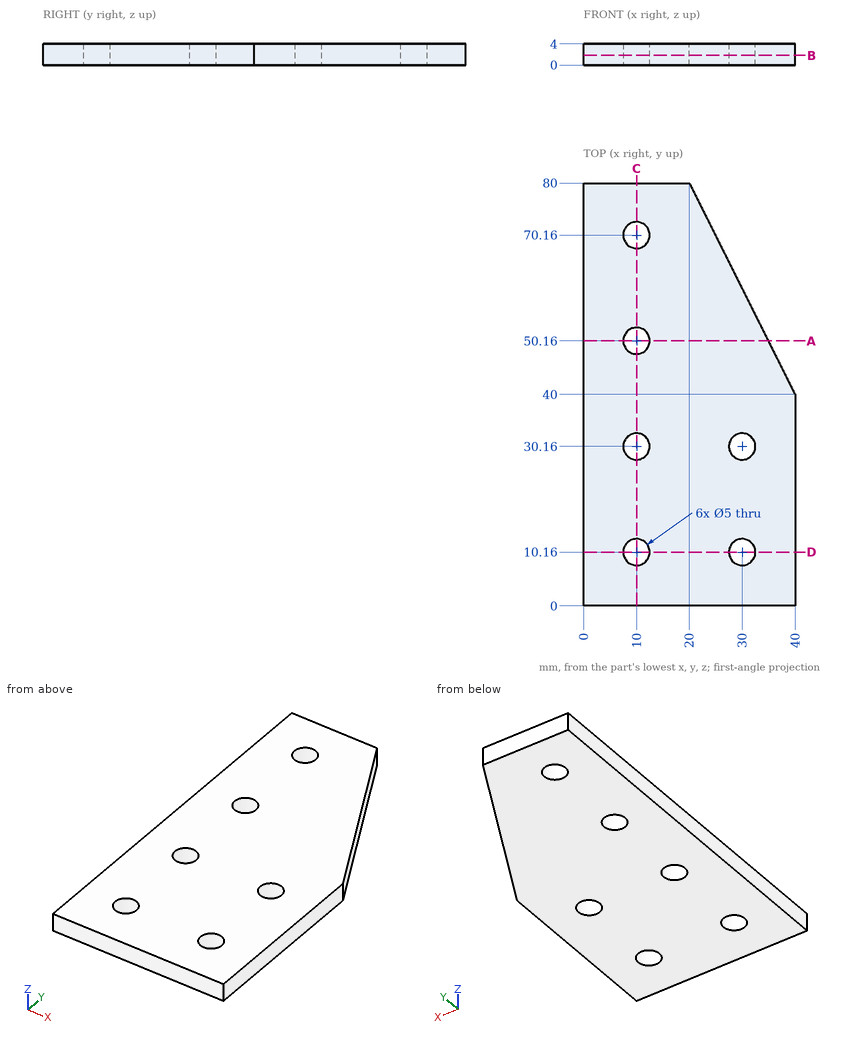
Verification items for this drawing (mm, ordinates from the low corner). Coordinates: 2 decimals unless noted, no trailing zeros. Write each loop counter-clockwise with the first axis right and the second up, starting at its lowest first coordinate (ties: lowest second). Pieces come first, ordered by that corner, then holes. Notation, with made-up numbers: M 43.5,32 L 86.5,32 A11 ccw 86.5,52 Z; hole C 43.5,43.5 d3. An arc over 180 degrees is marked long. Use CSV: the item, a comma, the result in double quotes.
Q1. Section check A-A, the plane y = 50.16. Enter the section's corners in (x, z).
Computed values:
outline,"M 0,0 L 7.5,0 L 7.5,4 L 0,4 Z; M 12.5,0 L 34.92,0 L 34.92,4 L 12.5,4 Z"
Q2. Thickness scan on line 1 along Y through (x, z) = (12, 2); line 2 along Y through (x, z) = (9, 0.3); line 3 along Y through (x, z) = (29, 1.65). Record the ranges inside material, lowest first. Write a range as [from, to].
Computed values:
line 1,"[0, 8.66], [11.66, 28.66], [31.66, 48.66], [51.66, 68.66], [71.66, 80]"
line 2,"[0, 7.87], [12.45, 27.87], [32.45, 47.87], [52.45, 67.87], [72.45, 80]"
line 3,"[0, 7.87], [12.45, 27.87], [32.45, 62]"
Q3. Section check B-B, the plane z = 1.85. Enter the section's corners in (x, y).
Computed values:
outline,"M 0,0 L 40,0 L 40,40 L 20,80 L 0,80 Z; hole C 10,10.16 d5; hole C 10,30.16 d5; hole C 10,50.16 d5; hole C 10,70.16 d5; hole C 30,10.16 d5; hole C 30,30.16 d5"
Q4. Section check D-D, the plane y = 10.16. Enter the section's corners in (x, z), and give its area (3 significant figures).
Computed values:
outline,"M 0,0 L 7.5,0 L 7.5,4 L 0,4 Z; M 12.5,0 L 27.5,0 L 27.5,4 L 12.5,4 Z; M 32.5,0 L 40,0 L 40,4 L 32.5,4 Z"
area,"120 mm²"
Q5. Section check C-C, the plane x = 10. Enter the section's corners in (y, z).
Computed values:
outline,"M 0,0 L 7.66,0 L 7.66,4 L 0,4 Z; M 12.66,0 L 27.66,0 L 27.66,4 L 12.66,4 Z; M 32.66,0 L 47.66,0 L 47.66,4 L 32.66,4 Z; M 52.66,0 L 67.66,0 L 67.66,4 L 52.66,4 Z; M 72.66,0 L 80,0 L 80,4 L 72.66,4 Z"
